Geometry check sheet. Reference: the model listing, model coordinates, mm. A direction names the side the tool comes from. Round coordinates to 2 decimals unless told otherwise and drop trailing zeros. Loops run counter-clockwise (first coordinate to the right, second up) from the corner with the lowest first, then second, coordinate; pieces in that order, holes last. Notation, with made-up numbers: (-26, 72) - (4, 72) arc R17 ccw to (4, 78) - close; hole circle Ø4 at (55.5, -6). An arc over 180 degrees is marked (long way). Answer in a Markdown table with one row per item. Add a question column.
Autodesk Inventor part; units mm, degrees
ref_plane "YZ Plane" through (0, 0, 0) normal (1, 0, 0) x (0, 1, 0)
ref_plane "XZ Plane" through (0, 0, 0) normal (0, 1, 0) x (-1, 0, 0)
ref_plane "XY Plane" through (0, 0, 0) normal (0, 0, 1) x (1, 0, 0)
sketch "Sketch16" plane through (0, 0, 0) normal (0, 0, 1) x (1, 0, 0)
  line L0 (0, 0) -> (-15.875, 0)
  line L1 (-15.875, -4.7625) -> (0, -4.7625)
  line L2 (0, 0) -> (0, -4.7625)
  line L3 (-15.875, -4.7625) -> (-15.875, 0)
  dimension "d96" = 15.875
  dimension "d184" = 4.7625
extrude "Extrusion17" add sketch "Sketch16" along normal blind 114.3
sketch "Sketch17" plane through (-15.875, 0, 0) normal (0, 1, 0) x (1, 0, 0)
  circle A0 centre (7.9375, -104.775) radius 6.5768
  line L0 (0, 0) -> (0, -114.3)
  line L1 (15.875, -114.3) -> (0, -114.3)
  circle A1 centre (7.9375, -88.9) radius 6.5768
  circle A2 centre (7.9375, -73.025) radius 6.5768
  circle A3 centre (7.9375, -57.15) radius 6.5768
  circle A4 centre (7.9375, -41.275) radius 6.5768
  circle A5 centre (7.9375, -25.4) radius 6.5768
  circle A6 centre (7.9375, -9.525) radius 6.5768
  point P0 (15.875, 0)
  dimension "d102" = 13.1536
  dimension "d103" = 7.9375
  dimension "d104" = 9.525
  dimension "d107" = 15.875
sketch "Sketch44" plane through (0, -4.7625, 0) normal (1, 0, 0) x (0, 0, -1)
  arc A0 (4.7625, 0) -> (0, 4.7625) centre (0, 0) ccw
  line L0 (0, 0) -> (4.7625, 0)
  line L1 (0, 4.7625) -> (0, 0)
  arc A1 (-114.3, 4.7625) -> (-119.0625, 0) centre (-114.3, 0) ccw
  line L2 (-114.3, 4.7625) -> (-114.3, 0)
  line L3 (-114.3, 0) -> (-119.0625, 0)
extrude "Extrusion40" add sketch "Sketch44" against normal up to surface (15.875 mm away)
ref_plane "Work Plane1" through (0, -4.7625, 119.0625) normal (0, 0, 1) x (1, 0, 0)
sketch "Sketch45" plane through (0, -4.7625, 119.0625) normal (0, 0, 1) x (1, 0, 0)
  line L0 (-15.875, 0) -> (-15.875, 4.7625)
  arc A0 (-15.875, 1.5875) -> (-15.875, 3.175) centre (-15.875, 2.3812) ccw
  line L1 (0, 4.7625) -> (0, 0)
  arc A1 (0, 3.175) -> (0, 1.5875) centre (0, 2.3813) ccw
  line L2 (-15.875, 3.175) -> (-15.875, 1.5875)
  line L3 (0, 3.175) -> (0, 1.5875)
  line L4 (0, 4.7625) -> (-15.875, 4.7625)
  dimension "d240" = 0.7937
  dimension "d241" = 0.7937
  dimension "d242" = 2.3813
  dimension "d243" = 2.3813
extrude "Extrusion41" cut sketch "Sketch45" against normal through all
extrude "Extrusion42" cut sketch "Sketch17" against normal blind 1.7859
properties part number "base"
Q1. Depth check by flat-ended pin: P1, Ø5, axis at x = -14, z = 14, coming from the +Y side; P2, Ø6.5, axis at x = -6.5, z = 9.5, coming from the +Y side. Enter the tip coordinate at first touch or a pass-through.
Q2. Cross-section at C-C, the plane z = 102. Enter the section's corners in (x, y) (1 decimal).
Q3. Release check for a two-part mould opening along Z. For faces 1 (the cylindrical face through (-7.83, -1.43, -3.4)), 2 (the cylindrical face through (-7.83, -1.36, 117.63)), 3 (the flat face through (-8, -1.786, 25)) record: +Z half, -Z half, draft (parallel to the pull), parting line (faces both ways), or undercut.
Q4. Set-up check for faces 4 (the flat face through (-8, -1.786, 89)), 5 (the flat face through (-1, 0, 56)): record each of +Z, -Z, +X, -X, +Y, -Y from which the full face is reachable in a straight line by a thin tool's end or side.
Q5. Cross-section at A-A, the plane z = 65. Enter the section's corners in (x, y) (1 decimal), plus the area to 3 significant figures.
Q6. Scan lines: line 1 (X direction, y = -1.15, z = 88.9) (3 decimals); line 2 (X direction, y = -2.5, z = 35.5); line 3 (Z direction, x = -5, y = -4.4). Record each from-to range of solid material in increasing order. Write a range as from..to.
Check sheet entries:
| question | item | result |
|---|---|---|
| 1 | P1 | y = 0 |
| 1 | P2 | y = -1.79 |
| 2 | outline | (-15.9, -4.8) - (0, -4.8) - (0, -3.2) arc R0.8 cw to (0, -1.6) - (0, 0) - (-2, 0) - (-2, -1.8) - (-13.9, -1.8) - (-13.9, 0) - (-15.9, 0) - (-15.9, -1.6) arc R0.8 cw to (-15.9, -3.2) - close |
| 3 | face 1 | -Z half |
| 3 | face 2 | +Z half |
| 3 | face 3 | undercut |
| 4 | face 4 | +Y |
| 4 | face 5 | +Z, -Z, +X, -X, +Y |
| 5 | outline | (-15.9, -4.8) - (0, -4.8) - (0, -3.2) arc R0.8 cw to (0, -1.6) - (0, 0) - (-15.9, 0) - (-15.9, -1.6) arc R0.8 cw to (-15.9, -3.2) - close |
| 5 | area | 73.6 mm² |
| 6 | line 1 | -15.875..-14.514, -1.361..0 |
| 6 | line 2 | -15.09..-0.78 |
| 6 | line 3 | -4.75..119.05 |
